from build123d import *

# Parameters (mm, degrees)
BOSS_EXTRUDE1_DEPTH = 5
FILLET2_R           = 5
FILLET3_R           = 5
FILLET4_R           = 5
FILLET5_R           = 5
FILLET6_R           = 5
FILLET7_R           = 5
FILLET8_R           = 5
FILLET9_R           = 5
SKETCH2_R           = 1.25
SKETCH2_R_2         = 2.5
SKETCH2_R_3         = 3
CUT_EXTRUDE1_DEPTH  = 10


with BuildPart() as part:
    # Sketch1 → Boss-Extrude1 (new body)
    with BuildSketch(Plane.XY):
        Polygon((21.15, 21.15), (41.15, 36.15), (111.15, 36.15), (111.15, -36.15), (41.15, -36.15), (21.15, -21.15), (-21.15, -21.15), (-21.15, 21.15), align=None)
    extrude(amount=BOSS_EXTRUDE1_DEPTH)

    # Fillet2
    fillet2_edges = [part.edges().sort_by_distance(p)[0] for p in [
        (-21.15, -21.15, 2.5),
    ]]
    fillet(fillet2_edges, radius=FILLET2_R)

    # Fillet3
    fillet3_edges = [part.edges().sort_by_distance(p)[0] for p in [
        (-21.15, 21.15, 2.5),
    ]]
    fillet(fillet3_edges, radius=FILLET3_R)

    # Fillet4
    fillet4_edges = [part.edges().sort_by_distance(p)[0] for p in [
        (21.15, 21.15, 2.5),
    ]]
    fillet(fillet4_edges, radius=FILLET4_R)

    # Fillet5
    fillet5_edges = [part.edges().sort_by_distance(p)[0] for p in [
        (21.15, -21.15, 2.5),
    ]]
    fillet(fillet5_edges, radius=FILLET5_R)

    # Fillet6
    fillet6_edges = [part.edges().sort_by_distance(p)[0] for p in [
        (41.15, -36.15, 2.5),
    ]]
    fillet(fillet6_edges, radius=FILLET6_R)

    # Fillet7
    fillet7_edges = [part.edges().sort_by_distance(p)[0] for p in [
        (41.15, 36.15, 2.5),
    ]]
    fillet(fillet7_edges, radius=FILLET7_R)

    # Fillet8
    fillet8_edges = [part.edges().sort_by_distance(p)[0] for p in [
        (111.15, 36.15, 2.5),
    ]]
    fillet(fillet8_edges, radius=FILLET8_R)

    # Fillet9
    fillet9_edges = [part.edges().sort_by_distance(p)[0] for p in [
        (111.15, -36.15, 2.5),
    ]]
    fillet(fillet9_edges, radius=FILLET9_R)

    # Sketch2 → Cut-Extrude1 (cut)
    with BuildSketch(Plane.XY.offset(5)):
        with Locations((-15.5, -15.5)):
            Circle(SKETCH2_R)
        with Locations((-15.5, 15.5)):
            Circle(SKETCH2_R)
        with Locations((15.5, 15.5)):
            Circle(SKETCH2_R)
        with Locations((15.5, -15.5)):
            Circle(SKETCH2_R)
        with Locations((106.15, 31.15)):
            Circle(SKETCH2_R_2)
        with Locations((106.15, -31.15)):
            Circle(SKETCH2_R_2)
        with Locations((43.95, -31.15)):
            Circle(SKETCH2_R_2)
        with Locations((43.95, 31.15)):
            Circle(SKETCH2_R_2)
        Circle(SKETCH2_R_3)
    extrude(amount=-CUT_EXTRUDE1_DEPTH, mode=Mode.SUBTRACT)


solid = part.part
Build history of the part. All positions in model axes, mm. A direction names the side the tool comes from. Give positions to 0.01 mm unless a question says otherwise; leave off trailing zeros. Write each loop counter-clockwise with the first axis right and the second up, starting at its lowest first coordinate (ties: lowest second). Pieces come first, ordered by that corner, then holes. Notation, with made-up numbers: (-22, 62.5) - (-13, 62.5) arc R27 cw to (-13, 86.5) - close; hole circle Ø3 at (57.25, 39). An arc over 180 degrees is marked (long way). Use one line per item in the form item = value. Start each with the question number.
1. Probe line 1 (Y direction, x = 15.5, z = 1.85); line 2 (Y direction, x = 45.5, z = 3.5); line 3 (Y direction, x = -14, z = 4.7). List the from-to ranges inside material, lowest first. Write a range as [from, to].
2. Band-saw the part on C-C on y = 0. Write the cut outline in (x, z).
3. Drop flat-ended pins along their axis: pin 1 Ø2.5 at (x, z) = (-5, 1.5) entering from -Y; pin 2 Ø1.5 at (y, z) = (25.5, 2) entering from -X. Give the stop position or say it passes through.
4. Two-plate mould, pull along Y, no slides. Class faces 1 (the face through (-15.66, -14.26, 2.54)), 2 (the face through (31.27, -28.74, 2.46)), 3 (the face through (41.26, 35.9, 2.54)), 4 (the face through (41.452, 31.26, 2.535)): released by +Y, released by -Y, zero draft, split by the parting line, or undercut.
5. Band-saw the part on B-B on x = 0. Write the cut outline in (y, z).
6. Band-saw the part on A-A on z = 2.2. Count the separate pieces of the cut face and the enclosed holes in it, plus the area to 3 significant figures.
7. 3-axis set-ups, long thin cutter, end or side, ignore diameter. For faces 5 (the face through (14.579, 16.345, 2.535)), 6 (the face through (1, 21.15, 2)): which of +Z, -Z, +X, -X, +Y, -Y reach the whole face in a straight line?
Conclusion:
q1.line_1 = [-21.15, -16.75], [-14.25, 14.25], [16.75, 21.15]
q1.line_2 = [-36.15, -33.11], [-29.19, 29.19], [33.11, 36.15]
q1.line_3 = [-21.15, 21.15]
q2.outline = (-21.15, 0) - (-3, 0) - (-3, 5) - (-21.15, 5) - close; (3, 0) - (111.15, 0) - (111.15, 5) - (3, 5) - close
q3.pin_1 = -21.15
q3.pin_2 = 25.95
q4.face_1 = undercut
q4.face_2 = released by -Y
q4.face_3 = released by +Y
q4.face_4 = undercut
q5.outline = (-21.15, 0) - (-3, 0) - (-3, 5) - (-21.15, 5) - close; (3, 0) - (21.15, 0) - (21.15, 5) - (3, 5) - close
q6.separate_pieces = 1
q6.enclosed_holes = 9
q6.area = 7,850 mm²
q7.face_5 = +Z, -Z
q7.face_6 = +Z, -Z, -X, +Y
